Geometry: final body of the model. Coordinates: model frame, mm. Give positions to 0.01 mm unless a question says otherwise; leave off trailing zeros. Loops run counter-clockwise (first coordinate to the right, second up) from the corner with the lowest first, then second, coordinate; pieces in that order, holes last. Notation, with made-up numbers: (-28, -31.75) - (-14, -31.75) arc R11 ccw to (-14, -14.75) - close; hole circle Ø6 at (-12.75, 36). An arc over 180 degrees is marked (long way). Use one line per item in the form item = value.
```python
from build123d import *

# Parameters (mm, degrees)
SKETCH1_R           = 2.5
BOSS_EXTRUDE1_DEPTH = 200
FILLET1_R           = 2


with BuildPart() as part:
    # Sketch1 → Boss-Extrude1 (new body)
    with BuildSketch(Plane.XY):
        Polygon((-5.46, -6.42), (-3.215, -4.175), (3.215, -4.175), (5.46, -6.42), (5.46, -8.22), (3.06, -8.22), (3.06, -10), (10, -10), (10, -3.06), (8.22, -3.06), (8.22, -5.46), (6.42, -5.46), (4.175, -3.215), (4.175, 3.215), (6.42, 5.46), (8.22, 5.46), (8.22, 3.06), (10, 3.06), (10, 10), (3.06, 10), (3.06, 8.22), (5.46, 8.22), (5.46, 6.42), (3.215, 4.175), (-3.215, 4.175), (-5.46, 6.42), (-5.46, 8.22), (-3.06, 8.22), (-3.06, 10), (-10, 10), (-10, 3.06), (-8.22, 3.06), (-8.22, 5.46), (-6.42, 5.46), (-4.175, 3.215), (-4.175, -3.215), (-6.42, -5.46), (-8.22, -5.46), (-8.22, -3.06), (-10, -3.06), (-10, -10), (-3.06, -10), (-3.06, -8.22), (-5.46, -8.22), align=None)
        Circle(SKETCH1_R, mode=Mode.SUBTRACT)
    extrude(amount=BOSS_EXTRUDE1_DEPTH)

    # Fillet1
    fillet1_edges = [part.edges().sort_by_distance(p)[0] for p in [
        (10, -10, 100),
        (-10, -10, 100),
        (-10, 10, 100),
        (10, 10, 100),
    ]]
    fillet(fillet1_edges, radius=FILLET1_R)


solid = part.part
```
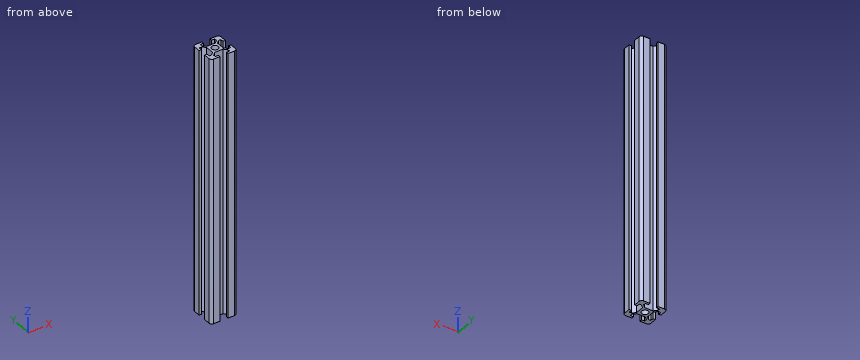
(1) Pin query (flat end, axial travel): P1, Ø3, axis at x = -1, z = 130, coming from the +Y side (3 decimals); P2, Ø0.5, axis at x = -9, z = 112, coming from the -Y side; P3, Ø0.9, axis at y = -9.5, z = 91.5, coming from the +X side. Return the tip coordinate at first contact, or that it passes through.
Solution:
P1 = 4.175
P2 = -9.85
P3 = 9.7
(2) Cut plane A-A (x = 0). Return the cut outline in (y, z) (3 decimals), plus the area to 3 significant figures.
Solution:
outline = (-4.175, 0) - (-2.5, 0) - (-2.5, 200) - (-4.175, 200) - close; (2.5, 0) - (4.175, 0) - (4.175, 200) - (2.5, 200) - close
area = 670 mm2
(3) Material intervals for L1, parallel to Y at x = 3.25, z = 71; L2, parallel to Y at x = 0, z = 56 (3 decimals); L3, parallel to X at y = 8.25, z = 57, sorted ascending. Write a range as from..to.
Solution:
L1 = -10..-8.22, -4.21..4.21, 8.22..10
L2 = -4.175..-2.5, 2.5..4.175
L3 = -9.98..-3.06, 3.06..9.98
